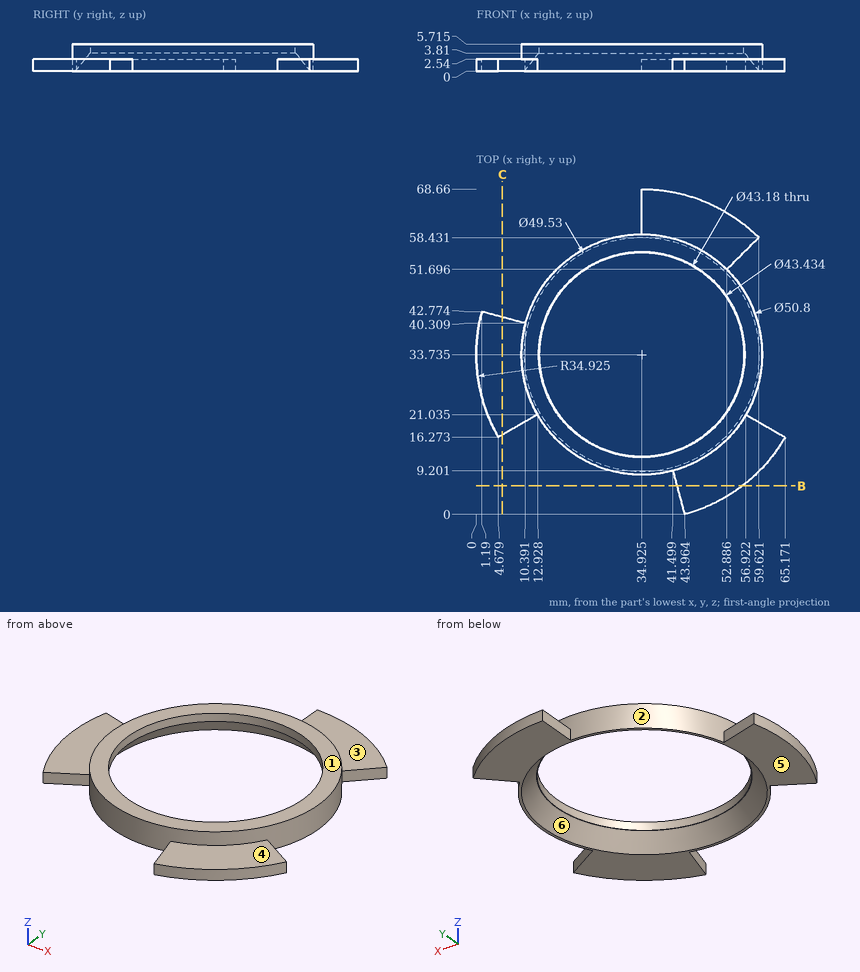
Geometry check sheet. Reference: drawing and pictorial views, mm from the part's lowest x, y, z. A direction names the side the tool comes from. Give positions to 0.01 mm unless a question says otherwise; leave off trailing zeros. Write each loop counter-clockwise with the first axis right and the second up, starting at its lowest first coordinate (ties: lowest second). Pieces come first, ordered by that corner, then holes. Notation, with made-up numbers: M 30,16 L 39,16 A16 ccw 39,41 Z; hole C 22.5,13 d3. An arc over 180 degrees is marked long. Answer as CSV lines item,"result". Start each with the question number.
Q1. Material ranges on L1, parallel to Y at x = 35, z = 3.9 (1 decimal); L2, parallel to Y at x = 35, z = 3.15 (1 decimal); L3, parallel to X at y = 16.5, z = 5.1 (1 decimal), recorded low to high.
Q2. Go/stop test with flat-tipped pins: pin 1 (1.5 mm diameter, centred on x = 15.5, y = 38.5, fed in from -Z); pin 2 (2 mm diameter, centred on y = 62.5, z = 2, fed in from -X) (1 decimal); pin 3 (1.5 mm diameter, centred on y = 10.5, z = 1, fed in from +X); pin 4 (5 mm diameter, centred on x = 48.5, y = 63.5, fed in from +Z). Record where each tip stops, or that it passes through.
Q3. Section check C-C, the plane x = 5.5. Record the cut outline in (y, z).
Q4. Section check B-B, the plane y = 6. Record the cut outline in (x, z).
Q5. Release check for a two-part mould opening along X. For the marked faces 5 and 6 record: pulls with the +X half, pulls with the -X half, needs draft (parallel to the pull), parting line crosses it, or undercut.
Q6. Tool access check on the marked faces 1, 2, 3 and 4. Record the directions out of +Z, -Z, +X, -X, +Y, -Y that give a thin tool (end or side, any length) a straight path to the whole face; none if there is none.
Geometry says:
1,L1,"8.3 to 12.1, 55.3 to 59.1"
1,L2,"8.3 to 11.5, 56 to 59.1"
1,L3,"16.3 to 21.9, 47.9 to 53.6"
2,pin 1,"through"
2,pin 2,"x = 34.9"
2,pin 3,"x = 61.65"
2,pin 4,"z = 2.54"
3,outline,"M 16.75,0 L 41.62,0 L 41.62,2.54 L 16.75,2.54 Z"
4,outline,"M 42.36,0 L 56.15,0 L 56.15,2.54 L 42.36,2.54 Z"
5,face 5,"needs draft"
5,face 6,"undercut"
6,face 1,"+Z, +X, -X, +Y, -Y"
6,face 2,"+Z"
6,face 3,"+Z, +X, +Y"
6,face 4,"+Z, +X, -Y"
